Here's how the part is built. I have some questions about the finished solid (model axes, mm). A direction names the side the tool comes from. Coordinates: 2 decimals unless noted, no trailing zeros. Write each loop counter-clockwise with the first axis right and the second up, starting at its lowest first coordinate (ties: lowest second). Pieces come first, ordered by that corner, then holes.
```python
from build123d import *

# Parameters (mm, degrees)
SKETCH1_R           = 4.25
BOSS_EXTRUDE1_DEPTH = 10
BOSS_EXTRUDE2_START = -5
BOSS_EXTRUDE2_DEPTH = 15
SKETCH3_W           = 102
SKETCH3_H           = 25
BOSS_EXTRUDE3_DEPTH = 224
CUT_EXTRUDE1_REACH  = 268.845
SKETCH4_R           = 5.75


with BuildPart() as part:
    # Sketch1 → Boss-Extrude1 (new body)
    with BuildSketch(Plane(origin=(0, 0, 0), x_dir=(1, 0, 0), z_dir=(0, 1, 0))):
        Polygon((-51, 11.25), (51, 11.25), (51, 0), (51, -13.75), (38, -13.75), (38, 0), (-38, 0), (-38, -13.75), (-51, -13.75), align=None)
        with Locations(Location((-44, 4.25, 0), (0, 0, 270))):
            Circle(SKETCH1_R, mode=Mode.SUBTRACT)
        with Locations(Location((44, 4.25, 0), (0, 0, 90))):
            Circle(SKETCH1_R, mode=Mode.SUBTRACT)
    boss_extrude1 = extrude(amount=BOSS_EXTRUDE1_DEPTH)

    # Sketch2 → Boss-Extrude2 (add)
    with BuildSketch(Plane.XY.offset(13.75).offset(BOSS_EXTRUDE2_START)):
        Polygon((-51, 85), (-51, 0), (-38, 0), (-38, 60), (38, 60), (38, 0), (51, 0), (51, 85), align=None)
    boss_extrude2 = extrude(amount=BOSS_EXTRUDE2_DEPTH)

    # Sketch3 → Boss-Extrude3 (add)
    with BuildSketch(Plane.XY.offset(23.75)):
        with Locations((0, 72.5)):
            Rectangle(SKETCH3_W, SKETCH3_H)
    extrude(amount=BOSS_EXTRUDE3_DEPTH)

    # Sketch4 → Cut-Extrude1 (cut, up to next)
    with BuildSketch(Plane(origin=(0, 85, 0), x_dir=(1, 0, 0), z_dir=(0, 1, 0)), mode=Mode.PRIVATE) as cut_extrude1_sk1:
        with Locations(Location((-26, -50.5, 0), (0, 0, 270))):
            Circle(SKETCH4_R)
    cut_extrude1_tool1 = extrude(cut_extrude1_sk1.sketch, amount=-CUT_EXTRUDE1_REACH, mode=Mode.PRIVATE) & part.part
    add(cut_extrude1_tool1.solids().sort_by_distance((-26, 85, 50.5))[0], mode=Mode.SUBTRACT)

    # Mirror3: Boss-Extrude2 across plane
    add(boss_extrude2.mirror(Plane(origin=(0, 0, 135.75), x_dir=(1, 0, 0), z_dir=(0, 0, -1))))

    # Mirror4: Boss-Extrude1 across plane
    add(boss_extrude1.mirror(Plane(origin=(0, 0, 135.75), x_dir=(1, 0, 0), z_dir=(0, 0, -1))))


solid = part.part
```
1) Will these pins go through, and if not, where does the flat tip stop? pin 1 (14.5 mm diameter, centred on x = 43.5, y = 38, fed in from -Z); pin 2 (4 mm diameter, centred on x = 45.5, y = 34.5, fed in from +Z); pin 3 (10 mm diameter, centred on x = -3, z = 191.5, fed in from -Y).
Values follow:
pin 1: stops at z = 8.75
pin 2: stops at z = 262.75
pin 3: stops at y = 60
2) Imagine slicing it at D-D on z = 275.75. Please give me the cut outline in (x, y).
Values follow:
outline: (-51, 0) - (-48.25, 0) - (-48.25, 10) - (-51, 10) - close; (-39.75, 0) - (39.75, 0) - (39.75, 10) - (-39.75, 10) - close; (48.25, 0) - (51, 0) - (51, 10) - (48.25, 10) - close
3) Imagine slicing it at B-B on y = 38. Please give me the cut outline in (x, z), then the cut area to 3 significant figures.
Values follow:
outline: (-51, 8.75) - (-38, 8.75) - (-38, 23.75) - (-51, 23.75) - close; (-51, 247.75) - (-38, 247.75) - (-38, 262.75) - (-51, 262.75) - close; (38, 8.75) - (51, 8.75) - (51, 23.75) - (38, 23.75) - close; (38, 247.75) - (51, 247.75) - (51, 262.75) - (38, 262.75) - close
area: 780 mm2
4) I need wall thicknesses on probe 1 along X at (y, z) = (7, -4.25); probe 2 along Z at (x, y) = (44, 7); probe 3 along X at (y, z) = (67, 50). Which ranges of each line are inside material? Lowest first, please.
Values follow:
probe 1: x = -51 to -48.25, -39.75 to 39.75, 48.25 to 51
probe 2: z = -11.25 to -8.5, 0 to 23.75, 247.75 to 271.5, 280 to 282.75
probe 3: x = -51 to -31.73, -20.27 to 51
5) Imagine slicing it at C-C on z = 50.5. Please give me the cut outline in (x, y).
Values follow:
outline: (-51, 60) - (-31.75, 60) - (-31.75, 85) - (-51, 85) - close; (-20.25, 60) - (51, 60) - (51, 85) - (-20.25, 85) - close
6) Imagine slicing it at A-A on x = -44. Please give me the cut outline in (y, z), then the cut area to 3 significant figures.
Values follow:
outline: (0, -11.25) - (10, -11.25) - (10, -8.5) - (0, -8.5) - close; (0, 0) - (10, 0) - (10, 8.75) - (85, 8.75) - (85, 262.75) - (10, 262.75) - (10, 271.5) - (0, 271.5) - (0, 247.75) - (60, 247.75) - (60, 23.75) - (0, 23.75) - close; (0, 280) - (10, 280) - (10, 282.75) - (0, 282.75) - close
area: 8,380 mm2
7) On a 3-axis mill with a long thin cutter (end or side, diameter ignored), from which of +Z, -Z, +X, -X, +Y, -Y can I reach the whole of each face in a straight line? I mean faces 1 (the face through (44, 30, 247.75)), 2 (the face through (-1, 65, 262.75)), 3 (the face through (1, 10, -4)). Say none if no direction works.
Values follow:
face 1: +X, -X, -Y
face 2: +Z, +X, -X, +Y
face 3: -Z, +X, -X, +Y
8) We'd pull the mould along X, two halves only. Please class faces 4 (the face through (-45, 30, 23.75)), 5 (the face through (51, 61, 135)), 6 (the face through (-38, 30, 257)): pulls with the +X half, pulls with the -X half, needs draft (parallel to the pull), parting line crosses it, or undercut.
Values follow:
face 4: needs draft
face 5: pulls with the +X half
face 6: undercut
